```python
from build123d import *

# Parameters (mm, degrees)
SKETCH1_W           = 40
SKETCH1_H           = 40
BOSS_EXTRUDE1_DEPTH = 40
CUT_EXTRUDE1_DEPTH  = 40
CUT_EXTRUDE2_DEPTH  = 20


with BuildPart() as part:
    # Sketch1 → Boss-Extrude1 (new body)
    with BuildSketch(Plane.XY):
        with Locations((20, 20)):
            Rectangle(SKETCH1_W, SKETCH1_H)
    extrude(amount=BOSS_EXTRUDE1_DEPTH)

    # Sketch2 → Cut-Extrude1 (cut)
    with BuildSketch(Plane.XY.offset(40)):
        Polygon((0, 0), (20, 40), (0, 40), align=None)
    extrude(amount=-CUT_EXTRUDE1_DEPTH, mode=Mode.SUBTRACT)

    # Sketch3 → Cut-Extrude2 (cut)
    with BuildSketch(Plane.XY.offset(40)):
        Polygon((20, 40), (20, 0), (0, 0), align=None)
    extrude(amount=-CUT_EXTRUDE2_DEPTH, mode=Mode.SUBTRACT)


solid = part.part
```
Check sheet for the modelled part. Datum: model origin and axes. Units: mm. A direction names the side the tool comes from. Give positions to 0.01 mm unless a question says otherwise; leave off trailing zeros. Loops run counter-clockwise (first coordinate to the right, second up) from the corner with the lowest first, then second, coordinate; pieces in that order, holes last. Notation, with made-up numbers: (31, -7) - (46, -7) arc R31 ccw to (46, 18) - close; hole circle Ø8 at (15, 18.25). An arc over 180 degrees is marked (long way). One line per question, with ' | ' between items. Start each with the question number.
1. Cross-section at C-C, the plane x = 12. Enter the section's corners in (y, z).
2. Cross-section at A-A, the plane y = 14. Enter the section's corners in (x, z).
3. Cross-section at D-D, the plane y = 24. Enter the section's corners in (x, z), plus the area to 3 significant figures.
4. Gauge pin test, flat ends, axial feed: pin 1 Ø10 at (x, y) = (13, 22) entering from +Z; pin 2 Ø1 at (x, z) = (5, 12.5) entering from +Y; pin 3 Ø3 at (y, z) = (13.5, 22.5) entering from -X. Record the tip position at first contact, or that the pin passes through.
5. Material ranges on line 1 along X through (y, z) = (22.5, 29.5); line 2 along Z through (x, y) = (12.5, 7); line 3 along X through (y, z) = (13, 6), recorded low to high. Write a range as [from, to].
6. Cross-section at B-B, the plane z = 8. Enter the section's corners in (x, y), plus the area to 3 significant figures.
7. Set-up check for faces 1 (the flat face through (20, 20, 30)), 2 (the flat face through (30, 40, 20)): record each of +Z, -Z, +X, -X, +Y, -Y from which the full face is reachable in a straight line by a thin tool's end or side.
Check result:
1) outline: (0, 0) - (24, 0) - (24, 20) - (0, 20) - close
2) outline: (7, 0) - (40, 0) - (40, 40) - (20, 40) - (20, 20) - (7, 20) - close
3) outline: (12, 0) - (40, 0) - (40, 40) - (20, 40) - (20, 20) - (12, 20) - close | area: 960 mm2
4) pin 1: stops at z = 20 | pin 2: stops at y = 11 | pin 3: stops at x = 20
5) line 1: x = [20, 40] | line 2: z = [0, 20] | line 3: x = [6.5, 40]
6) outline: (0, 0) - (40, 0) - (40, 40) - (20, 40) - close | area: 1,200 mm2
7) face 1: +Z, -X, +Y, -Y | face 2: +Z, -Z, +X, -X, +Y
